```python
from build123d import *

# Parameters (mm, degrees)
SKETCH3_W                = 10
SKETCH3_H                = 15
SKETCH3_R                = 1.75
BOSS_EXTRUDE1_DEPTH      = 2
BOSS_EXTRUDE1_2_DEPTH    = 2
BOSS_EXTRUDE2_DEPTH      = 1
BOSS_EXTRUDE2_DEPTH_BACK = 1
FILLET1_R                = 8


with BuildPart() as part:
    # Sketch3 → Boss-Extrude1 (new body)
    with BuildSketch(Plane(origin=(0, 0, 0), x_dir=(1, 0, 0), z_dir=(0, 1, 0))):
        with Locations((-17.609522653, -8.672957347)):
            Rectangle(SKETCH3_W, SKETCH3_H)
        with Locations(Location((-17.609522653, -8.672957347, 0), (0, 0, 270))):
            Circle(SKETCH3_R, mode=Mode.SUBTRACT)
    extrude(amount=BOSS_EXTRUDE1_DEPTH)



with BuildPart() as body_2:
    # Sketch3 → Boss-Extrude1 2 (new body)
    with BuildSketch(Plane(origin=(0, 0, 0), x_dir=(1, 0, 0), z_dir=(0, 1, 0))):
        with Locations((31.390477347, -8.672957347)):
            Rectangle(SKETCH3_W, SKETCH3_H)
        with Locations(Location((31.390477347, -8.672957347, 0), (0, 0, 270))):
            Circle(SKETCH3_R, mode=Mode.SUBTRACT)
    extrude(amount=BOSS_EXTRUDE1_2_DEPTH)


with BuildPart() as part_1:
    add(part.part)

    add(body_2.part)  # Boss-Extrude2 merges body 2
    # Sketch4 → Boss-Extrude2 (add, two sides: drawn at the far end of the back side and taken through both)
    with BuildSketch(Plane.XY.offset(8.672957347).offset(-BOSS_EXTRUDE2_DEPTH_BACK)):
        Polygon((-12.609522653, 2), (-12.609522653, 10), (26.390477347, 10), (26.390477347, 2), (28.390477347, 2), (28.390477347, 12), (-14.609522653, 12), (-14.609522653, 2), align=None)
    extrude(amount=BOSS_EXTRUDE2_DEPTH + BOSS_EXTRUDE2_DEPTH_BACK)

    # Fillet1
    # the kernel refuses this fillet: 8 mm, written as the material it adds along each edge
    with BuildSketch(Plane(origin=(26.390477347, 10, 7.672957347), x_dir=(0, -1, 0), z_dir=(0, 0, 1)), Plane(origin=(-12.609522653, 10, 7.672957347), x_dir=(1, 0, 0), z_dir=(0, 0, 1))) as fillet1_piece_1:
        with BuildLine():
            CenterArc((FILLET1_R, -FILLET1_R), FILLET1_R, 90, 90)
            Line((0, -FILLET1_R), (0, 0))
            Line((0, 0), (FILLET1_R, 0))
        make_face()
    extrude(amount=2)
    # the kernel refuses this fillet: 8 mm, written as the material it takes off along each edge
    with BuildSketch(Plane(origin=(-22.609522653, -20, 1.172957347), x_dir=(0, 0, 1), z_dir=(0, 1, 0)), Plane(origin=(36.390477347, -20, 1.172957347), x_dir=(-1, 0, 0), z_dir=(0, 1, 0)), Plane(origin=(36.390477347, -20, 16.172957347), x_dir=(0, 0, -1), z_dir=(0, 1, 0)), Plane(origin=(-14.609522653, 12, 29.672957347), x_dir=(1, 0, 0), z_dir=(0, 0, -1))) as fillet1_2_piece_1:
        with BuildLine():
            CenterArc((FILLET1_R, FILLET1_R), FILLET1_R, 180, 90)
            Line((0, FILLET1_R), (0, 0))
            Line((0, 0), (FILLET1_R, 0))
        make_face()
    extrude(amount=42, mode=Mode.SUBTRACT)
    with BuildSketch(Plane(origin=(-22.609522653, -20, 16.172957347), x_dir=(0, 0, -1), z_dir=(0, 1, 0)), Plane(origin=(28.390477347, 12, -12.327042653), x_dir=(0, -1, 0), z_dir=(0, 0, 1))) as fillet1_2_piece_2:
        with BuildLine():
            CenterArc((FILLET1_R, -FILLET1_R), FILLET1_R, 90, 90)
            Line((0, -FILLET1_R), (0, 0))
            Line((0, 0), (FILLET1_R, 0))
        make_face()
    extrude(amount=42, mode=Mode.SUBTRACT)


solid = part_1.part
```
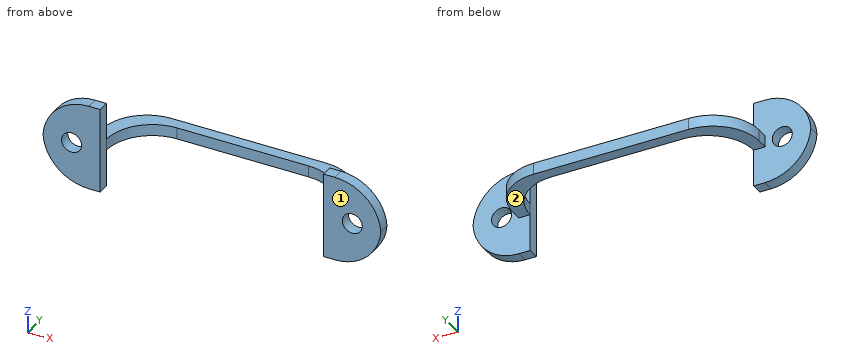
For this review, take the finished solid that the model builds, in its own axes (mm). Face numbers are marked on the shaded views. A direction names the side the tool comes from. Give positions to 0.01 mm unless a question says otherwise; leave off trailing zeros. Write each loop counter-clockwise with the first axis right and the second up, starting at its lowest first coordinate (ties: lowest second). Pieces come first, ordered by that corner, then holes. Notation, with made-up numbers: M 27.5,56 L 66.5,56 A12 ccw 66.5,64 Z; hole C 33.25,83 d4. An arc over 180 degrees is marked long. Answer as a JSON object with one key per item and string values. Group by question number.
Item 1: For pin 1 Ø2 at (y, z) = (8.5, 9) entering from +X; pin 2 Ø6 at (x, z) = (-12, 4.5) entering from -Y; pin 3 Ø4.5 at (x, z) = (31.39, 8.67) entering from +Y; pin 4 Ø6 at (y, z) = (3, 4.5) entering from -X, all flat-tipped, find the tip position at first contact; note any pin that passes through.
Item 2: Consider section A-A on z = 3.5. Write out the cut boundary in (x, y), plus the area to 3 significant figures.
Item 3: Tool access review of the marked faces 1 and 2: name each direction out of +Z, -Z, +X, -X, +Y, -Y from which nothing blocks a thin tool from reaching the whole face with its end or side.
Item 4: For probe 1 along Y at (x, z) = (-16, 10.5); probe 2 along X at (y, z) = (1, 5.75); probe 3 along Z at (x, y) = (-19, 1.25), list the stretches that pass through material, from the lowest coordinate up. Write a range as [from, to].
Item 5: Consider section D-D on y = 11. Write out the cut boundary in (x, z).
Item 6: Consider section B-B on y = 5. Write out the cut boundary in (x, z).
Item 7: Consider section C-C on x = -2.5. Write out the cut boundary in (y, z).
Check result:
{
 "1": {"pin 1": "stops at x = 27.58", "pin 2": "stops at y = 0", "pin 3": "stops at y = 2", "pin 4": "stops at x = -22.39"},
 "2": {"outline": "M -20.25,0 L -12.61,0 L -12.61,2 L -20.25,2 Z; M 26.39,0 L 34.03,0 L 34.03,2 L 26.39,2 Z", "area": "30.6 mm^2"},
 "3": {"face 1": "+Z, -Z, +X, -X, -Y", "face 2": "-Z, +X, -X, +Y"},
 "4": {"probe 1": "y = [0, 2]", "probe 2": "x = [-21.84, -12.61], [26.39, 35.62]", "probe 3": "z = [2.49, 7.61], [9.74, 14.86]"},
 "5": {"outline": "M -10.48,7.67 L 24.26,7.67 L 24.26,9.67 L -10.48,9.67 Z"},
 "6": {"outline": "M -14.55,7.67 L -12.03,7.67 L -12.03,9.67 L -14.55,9.67 Z; M 25.81,7.67 L 28.33,7.67 L 28.33,9.67 L 25.81,9.67 Z"},
 "7": {"outline": "M 10,7.67 L 12,7.67 L 12,9.67 L 10,9.67 Z"}
}
